from build123d import *

# Parameters (mm, degrees)
F0_W     = 1828.8
F0_H     = 914.4
F1_DEPTH = 660.4
F2_W     = 1625.6
F2_H     = 711.2
F3_DEPTH = 558.8
F4_R     = 12.7


with BuildPart() as f1:
    # F0 (on Top) → F1 (new body)
    with BuildSketch(Plane.XY):
        Rectangle(F0_W, F0_H)
    extrude(amount=F1_DEPTH)

    # F2 (on face) → F3 (cut)
    with BuildSketch(Plane.XY.offset(660.4)):
        Rectangle(F2_W, F2_H)
    extrude(amount=-F3_DEPTH, mode=Mode.SUBTRACT)

    # F4
    f4_edges = [f1.edges().sort_by_distance(p)[0] for p in [
        (0, -355.6, 101.6),
        (812.8, 0, 101.6),
        (0, 355.6, 101.6),
        (-812.8, 0, 101.6),
        (812.8, 355.6, 381),
        (-812.8, 355.6, 381),
        (0, 355.6, 660.4),
        (-812.8, -355.6, 381),
        (-812.8, 0, 660.4),
        (812.8, -355.6, 381),
        (812.8, 0, 660.4),
        (0, -355.6, 660.4),
        (-914.4, -457.2, 330.2),
        (914.4, -457.2, 330.2),
        (0, -457.2, 0),
        (0, -457.2, 660.4),
        (914.4, 457.2, 330.2),
        (914.4, 0, 0),
        (914.4, 0, 660.4),
        (-914.4, 457.2, 330.2),
        (0, 457.2, 0),
        (0, 457.2, 660.4),
        (-914.4, 0, 0),
        (-914.4, 0, 660.4),
    ]]
    fillet(f4_edges, radius=F4_R)


solid = f1.part
Check sheet for the modelled part. Datum: model origin and axes. Units: mm. A direction names the side the tool comes from. Round coordinates to 2 decimals unless told otherwise and drop trailing zeros. Write each loop counter-clockwise with the first axis right and the second up, starting at its lowest first coordinate (ties: lowest second). Pieces come first, ordered by that corner, then holes. Notation, with made-up numbers: (7, -11) -> (41, -11) arc R28 ccw to (41, 20) -> close; hole circle Ø8 at (-21.5, 30). An arc over 180 degrees is marked (long way). Answer as CSV lines item,"result". Start each with the question number.
1) Material ranges on line 1 (Y direction, x = -584.5, z = 405.5); line 2 (X direction, y = -229, z = 574); line 3 (Z direction, x = -686.5, y = 281), recorded low to high. Write a range as from..to.
2) Section check A-A on z = 565.5. Enter the section's corners in (x, y), and give its area (3 significant figures).
3) Section check B-B on x = -736.5. Enter the section's corners in (y, z), and give its area (3 significant figures).
4) Release check for a two-part mould opening along X. For faces 3 (the flat face through (-11, -355.6, 385)), 4 (the flat face through (-13, 6, 0)), 5 (the flat face through (-914.4, -6, 326)), 6 (the flat face through (914.4, -6, 326)) record: pulls with the +X half, pulls with the -X half, needs draft (parallel to the pull), parting line crosses it, or undercut.
5) Section check C-C on y = 206.5. Enter the section's corners in (x, z).
6) Go/stop test with a flat-tipped pin: P1, Ø4, axis at x = -663, y = 58, coming from the +Z side. Record where the tip stops, or that it passes through.
7) Tool access check on faces 1 (the flat face through (-71, -393, 660.4)), 2 (the flat face through (812.8, -5, 385)). Record the directions out of +Z, -Z, +X, -X, +Y, -Y that give a thin tool (end or side, any length) a straight path to the whole face; none if there is none.
Found:
1,line 1,"y = -457.2..-355.6, 355.6..457.2"
1,line 2,"x = -914.4..-812.8, 812.8..914.4"
1,line 3,"z = 0..101.6"
2,outline,"(-914.4, -444.5) arc R12.7 ccw to (-901.7, -457.2) -> (901.7, -457.2) arc R12.7 ccw to (914.4, -444.5) -> (914.4, 444.5) arc R12.7 ccw to (901.7, 457.2) -> (-901.7, 457.2) arc R12.7 ccw to (-914.4, 444.5) -> close; hole (-812.8, -342.9) arc R12.7 ccw to (-800.1, -355.6) -> (800.1, -355.6) arc R12.7 ccw to (812.8, -342.9) -> (812.8, 342.9) arc R12.7 ccw to (800.1, 355.6) -> (-800.1, 355.6) arc R12.7 ccw to (-812.8, 342.9) -> close"
2,area,"516,000 mm^2"
3,outline,"(-457.2, 12.7) arc R12.7 ccw to (-444.5, 0) -> (444.5, 0) arc R12.7 ccw to (457.2, 12.7) -> (457.2, 647.7) arc R12.7 ccw to (444.5, 660.4) -> (368.3, 660.4) arc R12.7 ccw to (355.6, 647.7) -> (355.6, 114.3) arc R12.7 cw to (342.9, 101.6) -> (-342.9, 101.6) arc R12.7 cw to (-355.6, 114.3) -> (-355.6, 647.7) arc R12.7 ccw to (-368.3, 660.4) -> (-444.5, 660.4) arc R12.7 ccw to (-457.2, 647.7) -> close"
3,area,"206,000 mm^2"
4,face 3,"undercut"
4,face 4,"needs draft"
4,face 5,"pulls with the -X half"
4,face 6,"pulls with the +X half"
5,outline,"(-914.4, 12.7) arc R12.7 ccw to (-901.7, 0) -> (901.7, 0) arc R12.7 ccw to (914.4, 12.7) -> (914.4, 647.7) arc R12.7 ccw to (901.7, 660.4) -> (825.5, 660.4) arc R12.7 ccw to (812.8, 647.7) -> (812.8, 114.3) arc R12.7 cw to (800.1, 101.6) -> (-800.1, 101.6) arc R12.7 cw to (-812.8, 114.3) -> (-812.8, 647.7) arc R12.7 ccw to (-825.5, 660.4) -> (-901.7, 660.4) arc R12.7 ccw to (-914.4, 647.7) -> close"
6,P1,"stops at z = 101.6"
7,face 1,"+Z, +X, -X, +Y, -Y"
7,face 2,"+Z"
